Verification items for the finished model (mm, model axes). Round coordinates to 2 decimals unless told otherwise and drop trailing zeros. Write each loop counter-clockwise with the first axis right and the second up, starting at its lowest first coordinate (ties: lowest second). Pieces come first, ordered by that corner, then holes. Notation, with made-up numbers: (-29.5, 55) - (-9.5, 55) arc R33 ccw to (-9.5, 91) - close; hole circle Ø8 at (-13, -5.5). An arc over 180 degrees is marked (long way). Answer as a JSON object with one key per item and string values.
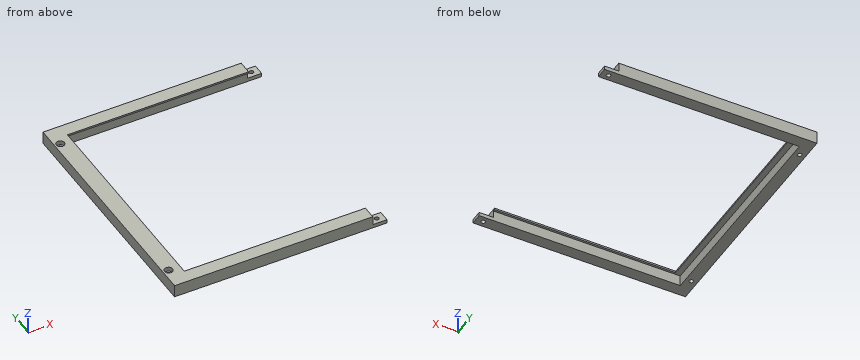
Autodesk Inventor part; units mm, degrees
ref_plane "YZ Plane" through (0, 0, 0) normal (1, 0, 0) x (0, 1, 0)
ref_plane "XZ Plane" through (0, 0, 0) normal (0, 1, 0) x (-1, 0, 0)
ref_plane "XY Plane" through (0, 0, 0) normal (0, 0, 1) x (1, 0, 0)
sketch "Skizze1" plane through (0, 0, 0) normal (0, 0, 1) x (1, 0, 0)
  line L0 (0, 0) -> (139.4, 0) construction
  line L1 (139.4, 0) -> (139.4, 169.5) construction
  line L2 (139.4, 169.5) -> (0, 169.5)
  line L3 (0, 169.5) -> (0, 0)
  line L4 (139.4, 160) -> (12, 160)
  line L5 (12, 160) -> (12, 9.5)
  line L6 (12, 9.5) -> (139.4, 9.5)
  line L7 (139.4, 9.5) -> (139.4, 160) construction
  line L8 (0, 0) -> (139.4, 0)
  line L9 (139.4, 0) -> (139.4, 9.5)
  line L10 (139.4, 160) -> (139.4, 169.5)
  dimension "d0" = 9.5
  dimension "d1" = 9.5
  dimension "d2" = 12
  dimension "d3" = 150.5
  dimension "d4" = 127.4
extrude "Extrusion1" add sketch "Skizze1" along normal blind 1.2
sketch "Skizze2" plane through (0, 0, 0) normal (0, 0, -1) x (-1, 0, 0)
  line L0 (-139.4, 8) -> (-8, 8)
  line L1 (-8, 8) -> (-8, 161.5)
  line L2 (-8, 161.5) -> (-139.4, 161.5)
  line L3 (0, 0) -> (-139.4, 0)
  line L4 (0, 0) -> (0, 169.5)
  line L5 (0, 169.5) -> (-139.4, 169.5)
  line L6 (-139.4, 160) -> (-139.4, 169.5)
  line L7 (-139.4, 169.5) -> (-149.4, 169.5)
  line L8 (-149.4, 169.5) -> (-149.4, 161.5)
  line L9 (-149.4, 161.5) -> (-139.4, 161.5)
  line L10 (-139.4, 0) -> (-139.4, 9.5)
  line L11 (-139.4, 0) -> (-149.4, 0)
  line L12 (-149.4, 0) -> (-149.4, 8)
  line L13 (-149.4, 8) -> (-139.4, 8)
  circle A0 centre (-144.4, 165.5) radius 1.5
  circle A1 centre (-144.4, 4) radius 1.5
  dimension "d7" = 10
  dimension "d8" = 8
  dimension "d9" = 8
  dimension "d10" = 8
  dimension "d11" = 3
  dimension "d12" = 5
  dimension "d13" = 4
  dimension "d14" = 3
  dimension "d15" = 5
  dimension "d16" = 4
extrude "Extrusion2" add sketch "Skizze2" along normal blind 7.7
sketch "Skizze3" plane through (0, 0, 0) normal (0, 0, 1) x (1, 0, 0)
  line L0 (139.4, 169.5) -> (139.4, 161.5)
  line L1 (139.4, 161.5) -> (149.4, 161.5)
  line L2 (149.4, 161.5) -> (149.4, 169.5)
  line L3 (149.4, 169.5) -> (139.4, 169.5)
  circle A0 centre (144.4, 165.5) radius 1.5
  line L4 (139.4, 8) -> (139.4, 0)
  line L5 (139.4, 0) -> (149.4, 0)
  line L6 (149.4, 0) -> (149.4, 8)
  line L7 (149.4, 8) -> (139.4, 8)
  circle A1 centre (144.4, 4) radius 1.5
  point P0 (0, 0)
extrude "Extrusion3" cut sketch "Skizze3" against normal blind 5.1
sketch "Skizze4" plane through (0, 0, 1.2) normal (0, 0, 1) x (1, 0, 0)
  line L0 (139.4, 169.5) -> (0, 169.5) construction
  line L1 (4, 169.5) -> (4, 0) construction
  line L2 (0, 0) -> (139.4, 0) construction
  line L3 (0, 169.5) -> (0, 0) construction
  circle A0 centre (4, 15) radius 2.85
  circle A1 centre (4, 154.5) radius 2.85
  dimension "d21" = 4
  dimension "d22" = 5.7
  dimension "d23" = 5.7
  dimension "d24" = 15
  dimension "d25" = 15
extrude "Extrusion4" cut sketch "Skizze4" against normal blind 3.1
sketch "Skizze5" plane through (4, 154.5, -1.9) normal (0, 0, 1) x (1, 0, 0)
  circle A0 centre (0, -139.5) radius 2.85
  circle A1 centre (0, 0) radius 2.85
  circle A2 centre (0, 0) radius 2.85
  circle A3 centre (0, 0) radius 1.5
  circle A4 centre (0, -139.5) radius 1.5
  point P0 (-4, -154.5)
  dimension "d28" = 3
  dimension "d29" = 3
extrude "Extrusion5" cut sketch "Skizze5" against normal blind 42.55 contours A3 | A4
equation "\"d1\" = d0"
equation "\"d14\" = d11"
equation "\"d22\" = d23"
equation "\"d25\" = d24"
equation "\"d28\" = d29"
properties part number "Case-Side"
1. Material ranges on probe 1 along Y at (x, z) = (23, -0.5); probe 2 along X at (y, z) = (4, -5.6); probe 3 along Y at (x, z) = (4, -0.6), recorded low to high. Write a range as from..to.
Completed:
{"probe 1": "y = 0..8, 161.5..169.5", "probe 2": "x = 0..142.9, 145.9..149.4", "probe 3": "y = 0..12.15, 17.85..151.65, 157.35..169.5"}
2. Cross-section at B-B (y = 36). Record the boundary of the cut face in (x, z), plus the area to 3 significant figures.
Completed:
{"outline": "(0, -7.7) - (8, -7.7) - (8, 0) - (12, 0) - (12, 1.2) - (0, 1.2) - close", "area": "76.0 mm^2"}
3. Cross-section at A-A (x = 38). Record the boundary of the cut face in (y, z), plus the area to 3 significant figures.
Completed:
{"outline": "(0, -7.7) - (8, -7.7) - (8, 0) - (9.5, 0) - (9.5, 1.2) - (0, 1.2) - close; (160, 0) - (161.5, 0) - (161.5, -7.7) - (169.5, -7.7) - (169.5, 1.2) - (160, 1.2) - close", "area": "146 mm^2"}
4. Go/stop test with flat-tipped pins: pin 1 (1.5 mm diameter, centred on y = 112.5, z = -5.5, fed in from +X); pin 2 (4 mm diameter, centred on x = 142, y = 4.5, fed in from +Z); pin 3 (3 mm diameter, centred on y = 4.5, z = -1.5, fed in from +X); pin 4 (5 mm diameter, centred on y = 149, z = -4, fed in from -X). Record where each tip stops, or that it passes through.
Completed:
{"pin 1": "stops at x = 8", "pin 2": "stops at z = -5.1", "pin 3": "stops at x = 139.4", "pin 4": "stops at x = 0"}
